Answer from the drawing. Dimensions are ordinates in mm from the lowest x, y and z of the part. A direction names the side the tool comes from. Round coordinates to 2 decimals unless told otherwise and drop trailing zeros. Order: outer loops, then holes, each group sorted by start corner. A loop starts at its lowest first (then second) coordinate and runs counter-clockwise, first axis right, second up.
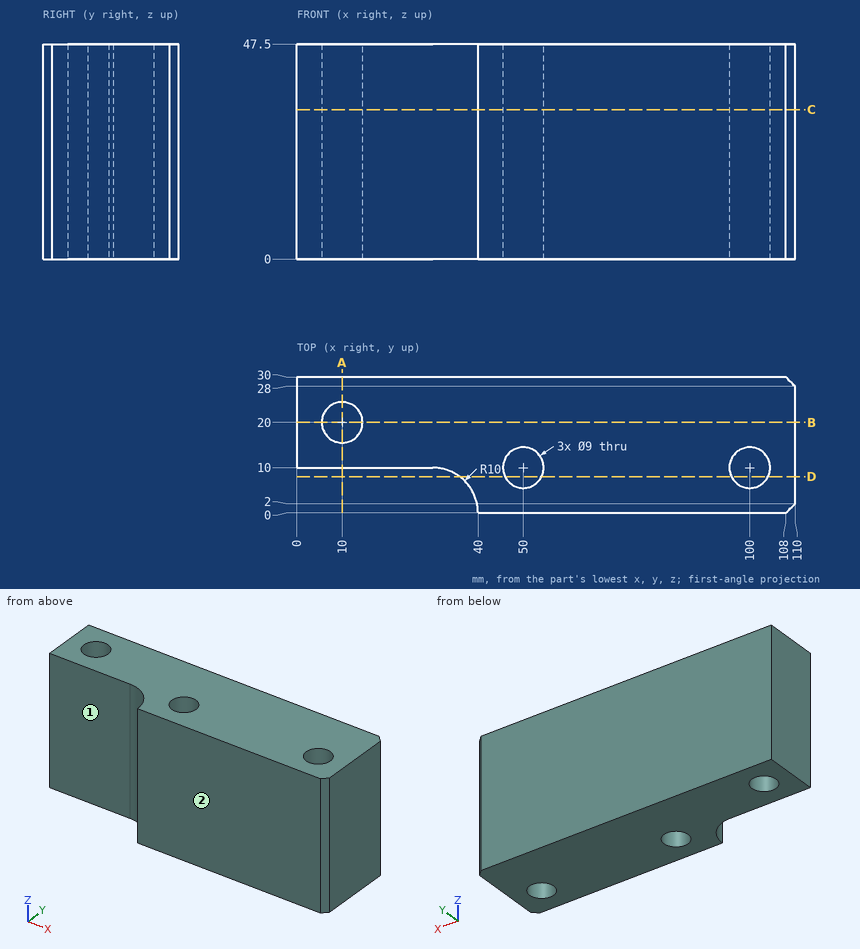
Q1. Straight lines are drawn through the part: probe 1 along Y at (x, z) = (100, 27); probe 2 along X at (y, z) = (7.75, 43.5); probe 3 along X at (y, z) = (6, 22.5). For each, find the intervals that lie inside material, in ascending order.
Outcome:
probe 1: y = 0 to 5.5, 14.5 to 30
probe 2: x = 36.32 to 46.1, 53.9 to 96.1, 103.9 to 110
probe 3: x = 38 to 47.94, 52.06 to 97.94, 102.06 to 110
Q2. Flat-ended cylindrical pins translate along their axes: pin 1 (6 mm diameter, centred on x = 31, z = 8, fed in from -Y) (3 decimals); pin 2 (8 mm diameter, centred on x = 50, y = 10, fed in from -Z); pin 3 (10 mm diameter, centred on x = 13, z = 18, fed in from -Y); pin 4 (5 mm diameter, centred on x = 28.5, z = 27.5, fed in from -Y). Find the tip coordinate at first contact, or state that the pin passes through.
Outcome:
pin 1: stops at y = 9.165
pin 2: passes through
pin 3: stops at y = 10
pin 4: stops at y = 9.95
Q3. A cutting plane is placed at A-A, the plane x = 10. Give the vertices of the cut face in (y, z), plus the area to 4 significant figures.
Outcome:
outline: (10, 0) - (15.5, 0) - (15.5, 47.5) - (10, 47.5) - close; (24.5, 0) - (30, 0) - (30, 47.5) - (24.5, 47.5) - close
area: 522.5 mm2
Q4. A cutting plane is placed at C-C, the plane z = 33. Give the number of separate pieces and of enclosed holes in the cut face, plus the area to 3 significant figures.
Outcome:
separate pieces: 1
enclosed holes: 3
area: 2,730 mm2
Q5. For the marked faces 1 and 2, determine the directions among +Z, -Z, +X, -X, +Y, -Y from which every point of the face is accessible in a straight line to the end or side of a thin tool.
Outcome:
face 1: +Z, -Z, -X, -Y
face 2: +Z, -Z, +X, -X, -Y
Q6. A cutting plane is placed at B-B, the plane y = 20. Give the vertices of the cut face in (x, z).
Outcome:
outline: (0, 0) - (5.5, 0) - (5.5, 47.5) - (0, 47.5) - close; (14.5, 0) - (110, 0) - (110, 47.5) - (14.5, 47.5) - close
Q7. A cutting plane is placed at D-D, the plane y = 8. Give the vertices of the cut face in (x, z), plus the area to 3 significant figures.
Outcome:
outline: (36, 0) - (45.97, 0) - (45.97, 47.5) - (36, 47.5) - close; (54.03, 0) - (95.97, 0) - (95.97, 47.5) - (54.03, 47.5) - close; (104.03, 0) - (110, 0) - (110, 47.5) - (104.03, 47.5) - close
area: 2,750 mm2
